from build123d import *

# Parameters (mm, degrees)
SKETCH1_W             = 28.575
SKETCH1_H             = 6.35
SKETCH2_R             = 14.2748
BOSS_EXTRUDE1_DEPTH   = 12.7
CUT_EXTRUDE1_DEPTH    = 45.676210112
F_8_CLEARANCE_HOLE1_D = 4.318


with BuildPart() as part:
    # Sketch1 → Revolve1 (revolve)
    with BuildSketch(Plane.XY):
        with Locations((14.2875, -3.175)):
            Rectangle(SKETCH1_W, SKETCH1_H)
    revolve(axis=Axis((0, 0, 0), (0, -1, 0)))

    # Sketch2 → Boss-Extrude1 (add)
    with BuildSketch(Plane.XZ.offset(6.35)):
        with Locations(Location((0, 0, 0), (0, 0, 180))):
            Circle(SKETCH2_R)
    extrude(amount=BOSS_EXTRUDE1_DEPTH)

    # Sketch3 → Cut-Extrude1 (cut, through all)
    with BuildSketch(Plane(origin=(0, 0, 0), x_dir=(-1, 0, 0), z_dir=(0, 1, 0))):
        Polygon((0, -7.347013116), (6.3627, -3.673506558), (6.3627, 3.673506558), (0, 7.347013116), (-6.3627, 3.673506558), (-6.3627, -3.673506558), align=None)
    extrude(amount=-CUT_EXTRUDE1_DEPTH, mode=Mode.SUBTRACT)

    # #8 Clearance Hole1 (through all)
    with Locations(Plane.XZ.offset(6.35)):
        with Locations((-20.622229928, -11.90625), (0, 23.8125), (0, -23.8125), (-20.622229928, 11.90625), (20.622229928, -11.90625)):
            Hole(F_8_CLEARANCE_HOLE1_D / 2)


solid = part.part
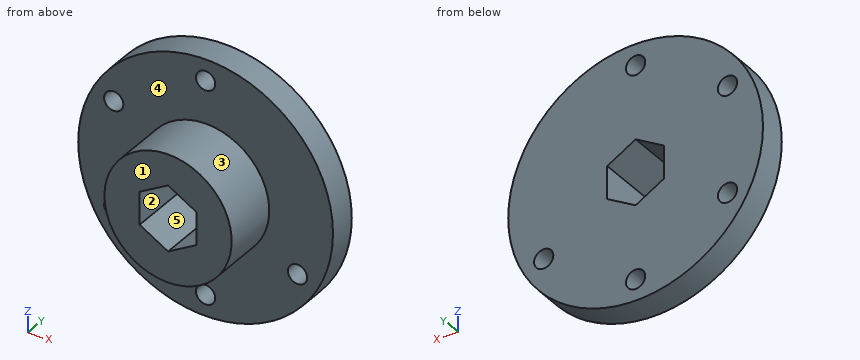
The model under review builds one solid part; all positions refer to its coordinate system, in mm. Face numbers are marked on the shaded views. A direction names the side the tool comes from. Coordinates: 2 decimals unless noted, no trailing zeros. Write each loop counter-clockwise with the first axis right and the second up, starting at its lowest first coordinate (ties: lowest second). Pieces come first, ordered by that corner, then holes. Notation, with made-up numbers: M 65.5,-36 L 112.5,-36 A23 cw 112.5,-18 Z; hole C 76.5,71.5 d10. An arc over 180 degrees is marked long. Put each result on its own line as item: value.
1) Draft analysis for pull direction Z (two halves, no side actions). For the marked faces 3, 4 and 5, state which applies: released by +Z, released by -Z, zero draft, split by the parting line, or undercut.
Computed:
face 3: split by the parting line
face 4: zero draft
face 5: undercut
2) For the marked faces 1 and 2, list the 3-axis set-ups (+Z, -Z, +X, -X, +Y, -Y) from which the entire face can be reached by the end or side of a thin tool; tool diameter is ignored.
Computed:
face 1: +Z, -Z, +X, -X, -Y
face 2: +Y, -Y
3) Add section D-D on x = 12. Give the boundary of the cut face in (y, z), then the cut area to 3 significant figures.
Computed:
outline: M -19.05,-7.73 L -6.35,-7.73 L -6.35,-25.93 L 0,-25.93 L 0,25.93 L -6.35,25.93 L -6.35,7.73 L -19.05,7.73 Z
area: 526 mm2
4) Add section B-B on z = 0. Give the boundary of the cut face in (x, y) (3 decimals), then the cut area to 3 significant figures.
Computed:
outline: M -28.575,-6.35 L -14.275,-6.35 L -14.275,-19.05 L -6.363,-19.05 L -6.363,0 L -28.575,0 Z; M 6.363,-19.05 L 14.275,-19.05 L 14.275,-6.35 L 28.575,-6.35 L 28.575,0 L 6.363,0 Z
area: 483 mm2
5) Clearance check with flat-ended pins moving along their axes: pin 1 Ø3 at (y, z) = (-3.5, -17.5) entering from +X; pin 2 Ø1 at (x, z) = (14.5, -21) entering from -Y; pin 3 Ø8 at (y, z) = (-7.5, 6) entering from +X; pin 4 Ø3.5 at (y, z) = (-8, 0.5) entering from -X (3 decimals). State where each tip first meets the part, or that it passes through.
Computed:
pin 1: stops at x = 23.68
pin 2: stops at y = -6.35
pin 3: stops at x = 28.49
pin 4: stops at x = -28.575
6) Add section C-C on x = -20. Give the boundary of the cut face in (y, z), then the cut area to 3 significant figures.
Computed:
outline: M -6.35,-20.41 L 0,-20.41 L 0,-13.97 L -6.35,-13.97 Z; M -6.35,-9.84 L 0,-9.84 L 0,9.84 L -6.35,9.84 Z; M -6.35,13.97 L 0,13.97 L 0,20.41 L -6.35,20.41 Z
area: 207 mm2
7) Add section A-A on y = -7.5. Give the boundary of the cut face in (x, z), then the cut area to 3 significant figures.
Computed:
outline: C 0,0 d28.55; hole M -6.36,-3.67 L 0,-7.35 L 6.36,-3.67 L 6.36,3.67 L 0,7.35 L -6.36,3.67 Z
area: 500 mm2
8) Wall thickness on probe 1 along Y at (x, z) = (22.5, 2); probe 2 along Z at (x, y) = (19.5, -5.5): over which ranges is each line inside the solid? List them lowest first. Write a range as [from, to].
Computed:
probe 1: y = [-6.35, 0]
probe 2: z = [-20.89, -13.75], [-10.06, 20.89]
